```python
from build123d import *

# Parameters (mm, degrees)
SKETCH1_W               = 70
SKETCH1_H               = 86
BOSS_EXTRUDE1_DEPTH     = 5
SKETCH2_W               = 12
SKETCH2_H               = 86
BOSS_EXTRUDE2_DEPTH     = 87
SKETCH4_R               = 38
CUT_EXTRUDE2_DEPTH      = 3
SKETCH5_R               = 2.6
CUT_EXTRUDE3_DEPTH      = 13
FILLET1_R               = 3
SKETCH6_R               = 20
CUT_EXTRUDE4_DEPTH      = 13
SKETCH7_W               = 12
SKETCH7_H               = 87
CUT_EXTRUDE5_DEPTH      = 87
FILLET2_R               = 1
BOSS_EXTRUDE4_DEPTH     = 8
SKETCH3_R               = 3
CUT_EXTRUDE1_DEPTH      = 14
SKETCH8_R               = 1.65
CUT_EXTRUDE6_DEPTH      = 9
CUT_EXTRUDE6_DEPTH_BACK = 6
SKETCH9_R               = 2.5
CUT_EXTRUDE7_DEPTH      = 14
SKETCH14_R              = 6.5
CUT_EXTRUDE8_DEPTH      = 8


with BuildPart() as part:
    # Sketch1 → Boss-Extrude1 (new body)
    with BuildSketch(Plane(origin=(0, 0, 0), x_dir=(1, 0, 0), z_dir=(0, 1, 0))):
        with Locations((35, -43)):
            Rectangle(SKETCH1_W, SKETCH1_H)
    extrude(amount=BOSS_EXTRUDE1_DEPTH)

    # Sketch2 → Boss-Extrude2 (add)
    with BuildSketch(Plane(origin=(0, 5, 0), x_dir=(1, 0, 0), z_dir=(0, 1, 0))):
        with Locations((64, -43)):
            Rectangle(SKETCH2_W, SKETCH2_H)
    extrude(amount=BOSS_EXTRUDE2_DEPTH)

    # Sketch4 → Cut-Extrude2 (cut)
    with BuildSketch(Plane.ZY.offset(-58)):
        with Locations((43, 56)):
            Circle(SKETCH4_R)
    extrude(amount=-CUT_EXTRUDE2_DEPTH, mode=Mode.SUBTRACT)

    # Sketch5 → Cut-Extrude3 (cut, through all)
    with BuildSketch(Plane.ZY.offset(-58)):
        with Locations((77.8, 90.8)):
            Circle(SKETCH5_R)
        with Locations((77.8, 21.2)):
            Circle(SKETCH5_R)
        with Locations((8.2, 90.8)):
            Circle(SKETCH5_R)
        with Locations((8.2, 21.2)):
            Circle(SKETCH5_R)
    extrude(amount=-CUT_EXTRUDE3_DEPTH, mode=Mode.SUBTRACT)

    # Fillet1
    fillet1_edges = [part.edges().sort_by_distance(p)[0] for p in [
        (64, 92, 0),
        (64, 92, 86),
    ]]
    fillet(fillet1_edges, radius=FILLET1_R)

    # Sketch6 → Cut-Extrude4 (cut, through all)
    with BuildSketch(Plane.ZY.offset(-58)):
        with Locations((43, 56)):
            Circle(SKETCH6_R)
    extrude(amount=-CUT_EXTRUDE4_DEPTH, mode=Mode.SUBTRACT)

    # Sketch7 → Cut-Extrude5 (cut, through all)
    with BuildSketch(Plane.XY.offset(86)):
        with Locations((64, 48.5)):
            Rectangle(SKETCH7_W, SKETCH7_H)
    extrude(amount=-CUT_EXTRUDE5_DEPTH, mode=Mode.SUBTRACT)

    # Fillet2
    fillet2_edges = [part.edges().sort_by_distance(p)[0] for p in [
        (0, 2.5, 0),
        (0, 2.5, 86),
        (70, 2.5, 0),
        (70, 2.5, 86),
    ]]
    fillet(fillet2_edges, radius=FILLET2_R)

    # Sketch12 → Boss-Extrude4 (add)
    with BuildSketch(Plane.XZ):
        with BuildLine():
            Line((70, 1), (70, 85))
            ThreePointArc((70, 85), (69.707106781, 85.707106781), (69, 86))
            Line((69, 86), (1, 86))
            ThreePointArc((1, 86), (0.292893219, 85.707106781), (0, 85))
            Line((0, 85), (0, 1))
            ThreePointArc((0, 1), (0.292893219, 0.292893219), (1, 0))
            Line((1, 0), (69, 0))
            ThreePointArc((69, 0), (69.707106781, 0.292893219), (70, 1))
        make_face()
    extrude(amount=BOSS_EXTRUDE4_DEPTH)

    # Sketch3 → Cut-Extrude1 (cut, through all)
    with BuildSketch(Plane(origin=(0, 5, 0), x_dir=(1, 0, 0), z_dir=(0, 1, 0))):
        with Locations((14, -8.4)):
            Circle(SKETCH3_R)
        with Locations((14, -77.6)):
            Circle(SKETCH3_R)
    extrude(amount=-CUT_EXTRUDE1_DEPTH, mode=Mode.SUBTRACT)

    # Sketch8 → Cut-Extrude6 (cut, two sides)
    with BuildSketch(Plane.XZ) as cut_extrude6_sk:
        with Locations((45, 68)):
            Circle(SKETCH8_R)
        with Locations((45, 18)):
            Circle(SKETCH8_R)
    extrude(amount=CUT_EXTRUDE6_DEPTH, mode=Mode.SUBTRACT)
    extrude(cut_extrude6_sk.sketch, amount=-CUT_EXTRUDE6_DEPTH_BACK, mode=Mode.SUBTRACT)

    # Sketch9 → Cut-Extrude7 (cut, through all)
    with BuildSketch(Plane(origin=(0, 5, 0), x_dir=(1, 0, 0), z_dir=(0, 1, 0))):
        with Locations((64, -10)):
            Circle(SKETCH9_R)
        with Locations((64, -76)):
            Circle(SKETCH9_R)
        with Locations((34, -70)):
            Circle(SKETCH9_R)
        with Locations((34, -16)):
            Circle(SKETCH9_R)
    extrude(amount=-CUT_EXTRUDE7_DEPTH, mode=Mode.SUBTRACT)

    # Sketch14 → Cut-Extrude8 (cut)
    with BuildSketch(Plane(origin=(0, 5, 0), x_dir=(1, 0, 0), z_dir=(0, 1, 0))):
        with Locations((14, -8.4)):
            Circle(SKETCH14_R)
        with Locations((14, -77.6)):
            Circle(SKETCH14_R)
    extrude(amount=-CUT_EXTRUDE8_DEPTH, mode=Mode.SUBTRACT)


solid = part.part
```
The model under review builds one solid part; all positions refer to its coordinate system, in mm. A direction names the side the tool comes from. Round coordinates to 2 decimals unless told otherwise and drop trailing zeros. Loops run counter-clockwise (first coordinate to the right, second up) from the corner with the lowest first, then second, coordinate; pieces in that order, holes last. Notation, with made-up numbers: (67.5, 49.25) - (84.5, 49.25) arc R27 cw to (84.5, 79.25) - close; hole circle Ø4 at (59, -8.5). An arc over 180 degrees is marked (long way). Use a Markdown table: item, result. Add a question column.
Q1. Add section C-C (x = 65.5). State the section outline as (y, z) points.
Q2. Add section B-B (y = -1.25). State how many separate pieces and enclosed holes the cut face has, plus the area to 3 significant figures.
Q3. The part is to be moulded in two halves that separate along X. For faces 1 (the face through (70, -1, 42)), 2 (the face through (35, -1, 0)), 3 (the face through (17, -3, 10)), say which applies: pulls with the +X half, pulls with the -X half, needs draft (parallel to the pull), parting line crosses it, or undercut.
Q4. For probe 1 along Z at (x, y) = (14, 4.5); probe 2 along Z at (x, y) = (14, -6.25); probe 3 along X at (y, z) = (0.25, 76), list the stretches that pass through material, from the lowest coordinate up.
Q5. Add section A-A (x = 14). State the section outline as (y, z) points, plus the area to 3 significant figures.
Q6. Add section D-D (z = 8.4). State the section outline as (x, y) points, plus the area to 3 significant figures.
Q7. Insertion check: pin 1 Ø4.5 at (x, z) = (64, 76) entering from +Y; pin 2 Ø4 at (x, z) = (12, 9.5) entering from +Y. Each pin has a flat end and moves straight along its axis. Give the tip position at first contact, or say it passes through.
Q8. Machinability: for faces 4 (the face through (13.154, 1.056, 71.155)), 5 (the face through (11.79, -5.46, 75.57)), which of the approach directions +Z, -Z, +X, -X, +Y, -Y give a long, thin tool a straight path to every point of the face, cutting with its end or side? Answer none if there is none.
Worked answers:
| question | item | result |
|---|---|---|
| 1 | outline | (-8, 0) - (5, 0) - (5, 8) - (-8, 8) - close; (-8, 12) - (5, 12) - (5, 74) - (-8, 74) - close; (-8, 78) - (5, 78) - (5, 86) - (-8, 86) - close |
| 2 | separate pieces | 1 |
| 2 | enclosed holes | 8 |
| 2 | area | 5,660 mm² |
| 3 | face 1 | pulls with the +X half |
| 3 | face 2 | needs draft |
| 3 | face 3 | undercut |
| 4 | probe 1 | 0 to 1.9, 14.9 to 71.1, 84.1 to 86 |
| 4 | probe 2 | 0 to 5.4, 11.4 to 74.6, 80.6 to 86 |
| 4 | probe 3 | 0 to 7.7, 20.3 to 61.5, 66.5 to 70 |
| 5 | outline | (-8, 0) - (5, 0) - (5, 1.9) - (-3, 1.9) - (-3, 5.4) - (-8, 5.4) - close; (-8, 11.4) - (-3, 11.4) - (-3, 14.9) - (5, 14.9) - (5, 71.1) - (-3, 71.1) - (-3, 74.6) - (-8, 74.6) - close; (-8, 80.6) - (-3, 80.6) - (-3, 84.1) - (5, 84.1) - (5, 86) - (-8, 86) - close |
| 5 | area | 850 mm² |
| 6 | outline | (0, -8) - (11, -8) - (11, -3) - (7.5, -3) - (7.5, 5) - (0, 5) - close; (17, -8) - (62.08, -8) - (62.08, 5) - (20.5, 5) - (20.5, -3) - (17, -3) - close; (65.92, -8) - (70, -8) - (70, 5) - (65.92, 5) - close |
| 6 | area | 726 mm² |
| 7 | pin 1 | through |
| 7 | pin 2 | y = -3 |
| 8 | face 4 | +Y |
| 8 | face 5 | +Y, -Y |
